Model file for the job. Use its own axes, mm. A direction names the side the tool comes from. Round coordinates to 2 decimals unless told otherwise and drop trailing zeros. Order: outer loops, then holes, each group sorted by start corner. A loop starts at its lowest first (then second) coordinate and runs counter-clockwise, first axis right, second up. Notation, with made-up numbers: (-1, 24.25) -> (7, 24.25) arc R18 cw to (7, 29.25) -> close; hole circle Ø4 at (67, -6.5). An arc over 180 degrees is marked (long way). Answer as CSV lines item,"result".
```python
from build123d import *

# Parameters (mm, degrees)
SKETCH2_W               = 3.590975848
SKETCH2_H               = 1.5
SKETCH2_W_2             = 2.734034887
SKETCH3_R               = 10
CUT_EXTRUDE1_DEPTH      = 24
SKETCH4_R               = 13
CUT_EXTRUDE2_DEPTH      = 10
CUT_EXTRUDE3_DEPTH      = 38.576588456
CUT_EXTRUDE3_DEPTH_BACK = 38.576588456
SKETCH5_R               = 2.5


with BuildPart() as part:
    # Sketch1 → Revolve1 (revolve)
    with BuildSketch(Plane.XY, mode=Mode.PRIVATE) as revolve1_sk:
        with BuildLine():
            Line((0, 0), (16, 0))
            Line((16, 0), (16, 27.795794509))
            Line((16, 27.795794509), (7, 29.382737335))
            ThreePointArc((7, 29.382737335), (3.513581264, 29.845385513), (0, 30))
            Line((0, 30), (0, 0))
        make_face()
    revolve(revolve1_sk.sketch.rotate(Axis((0, 30, 0), (0, -1, 0)), 180), axis=Axis((0, 30, 0), (0, -1, 0)))

    # Sketch2 → Cut-Revolve1 (revolve, cut)
    with BuildSketch(Plane.XY, mode=Mode.PRIVATE) as cut_revolve1_sk:
        with Locations((16.295487924, 26.25)):
            Rectangle(SKETCH2_W, SKETCH2_H)
        with Locations((15.867017443, 21.75)):
            Rectangle(SKETCH2_W_2, SKETCH2_H)
    revolve(cut_revolve1_sk.sketch.rotate(Axis((0, 0, 0), (0, 1, 0)), 90), axis=Axis((0, 0, 0), (0, 1, 0)), mode=Mode.SUBTRACT)

    # Sketch3 → Cut-Extrude1 (cut)
    with BuildSketch(Plane.XZ):
        Circle(SKETCH3_R)
    extrude(amount=-CUT_EXTRUDE1_DEPTH, mode=Mode.SUBTRACT)

    # Sketch4 → Cut-Extrude2 (cut)
    with BuildSketch(Plane(origin=(0, 0, 0), x_dir=(-1, 0, 0), z_dir=(0, -1, 0))):
        with Locations(Location((0, 0, 0), (0, 0, 180))):
            Circle(SKETCH4_R)
    extrude(amount=-CUT_EXTRUDE2_DEPTH, mode=Mode.SUBTRACT)

    # Sketch5 → Cut-Extrude3 (cut, two sides: drawn at the far end of the back side and taken through both)
    with BuildSketch(Plane(origin=(0, 0, 0), x_dir=(0, 0, -1), z_dir=(1, 0, 0)).offset(-CUT_EXTRUDE3_DEPTH_BACK)):
        with Locations(Location((0, 12, 0), (0, 0, 306.869897646))):
            Circle(SKETCH5_R)
    extrude(amount=CUT_EXTRUDE3_DEPTH + CUT_EXTRUDE3_DEPTH_BACK, mode=Mode.SUBTRACT)


solid = part.part
```
Q1. Tool access for faces 1 (the cylindrical face through (-14.78, 10.65, 6.13)), 2 (the flat face through (0, 24, 0)), 3 (the cylindrical face through (12.864, 26.26, -6.691)): list every direction of +Z, -Z, +X, -X, +Y, -Y with a clear straight run to the whole face (end or side of a thin tool).
Checks:
face 1,"+Y, -Y"
face 2,"-Y"
face 3,"none"
Q2. Mould opens along Y. For faces 4 (the cylindrical face through (3.47, 24.02, 15.62)), 5 (the flat face through (-14.3, 25.5, -3.6)), 6 (the flat face through (0.9, 10, 10.3)), 7 (the cylindrical face through (12.797, 14.488, -0.246)) say: +Y half, -Y half, draft (parallel to the pull), parting line (faces both ways), or undercut.
Checks:
face 4,"draft"
face 5,"undercut"
face 6,"-Y half"
face 7,"undercut"
Q3. Saw through at C-C (y = 12). Write the cut outline in (x, z), plus the area to 3 significant figures.
Checks:
outline,"(-15.8, -2.5) arc R16 ccw to (15.8, -2.5) -> (9.68, -2.5) arc R10 cw to (-9.68, -2.5) -> close; (-15.8, 2.5) -> (-9.68, 2.5) arc R10 cw to (9.68, 2.5) -> (15.8, 2.5) arc R16 ccw to start"
area,"430 mm²"
Q4. Saw through at D-D (y = 17.5). Write the cut outline in (x, z).
Checks:
outline,"circle Ø32 at (0, 0); hole circle Ø20 at (0, 0)"
Q5. Flat gauge pins, fed straight in: pin 1 (5 mm diameter, centred on x = -5.5, z = 4, fed in from +Y); pin 2 (12 mm diameter, centred on x = -8.5, z = -2, fed in from -Y); pin 3 (10 mm diameter, centred on x = -6.5, y = 9, fed in from -Z); pin 4 (9.5 mm diameter, centred on x = 7, z = 6.5, fed in from +Y). Where does each tip first touch, or does it go through?
Checks:
pin 1,"y = 29.77"
pin 2,"y = 0"
pin 3,"z = -15.93"
pin 4,"y = 29.71"
Q6. Saw through at A-A (z = 0). State how many separate pieces and enclosed holes the cut face has, plus the area to 3 significant figures.
Checks:
separate pieces,"3"
enclosed holes,"0"
area,"326 mm²"
Q7. Wall check: L1, parallel to Z at x = 0, y = 5; L2, parallel to Y at x = -9, z = 11.5; L3, parallel to X at y = 23.5, z = -4. Give the ranges that are in metal, low to high. Write a range as [from, to].
Checks:
L1,"[-16, -13], [13, 16]"
L2,"[0, 21], [22.5, 25.5], [27, 28.04]"
L3,"[-15.49, -9.17], [9.17, 15.49]"
